Read the model definition and answer for the solid it produces. Units are mm, in the model's axes. Face numbers are marked on the shaded views. A direction names the side the tool comes from. Give positions to 0.01 mm unless a question says otherwise; leave off trailing zeros. Write each loop counter-clockwise with the first axis right and the second up, starting at its lowest first coordinate (ties: lowest second). Pieces come first, ordered by that corner, then holes. Notation, with made-up numbers: (-26, 4) - (-4, 4) arc R23 ccw to (-4, 28) - close; hole circle Ø6 at (-5.75, 2.5). An arc over 180 degrees is marked (long way). Answer as a JSON object with one key per item and string values. Group by question number.
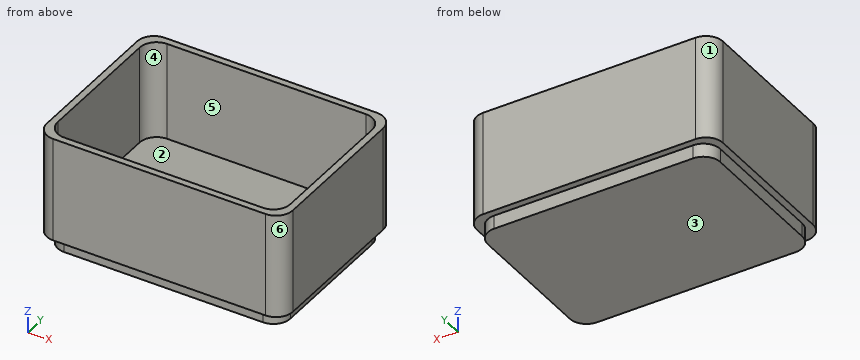
```python
from build123d import *

# Parameters (mm, degrees)
F1_DEPTH = 6
F2_DEPTH = 35
F3_DEPTH = 4


with BuildPart() as f1:
    # F0 (on Top) → F1 (new body)
    with BuildSketch(Plane.XY):
        with BuildLine():
            Line((31.5, 26.5), (-31.5, 26.5))
            ThreePointArc((-31.5, 26.5), (-35.0355339059, 25.0355339059), (-36.5, 21.5))
            Line((-36.5, 21.5), (-36.5, -21.5))
            ThreePointArc((-36.5, -21.5), (-35.0355339059, -25.0355339059), (-31.5, -26.5))
            Line((-31.5, -26.5), (31.5, -26.5))
            ThreePointArc((31.5, -26.5), (35.0355339059, -25.0355339059), (36.5, -21.5))
            Line((36.5, -21.5), (36.5, 21.5))
            ThreePointArc((36.5, 21.5), (35.0355339059, 25.0355339059), (31.5, 26.5))
        make_face()
        with BuildLine():
            ThreePointArc((-34.5, 19.5), (-33.0355339059, 23.0355339059), (-29.5, 24.5))
            Line((-29.5, 24.5), (29.5, 24.5))
            ThreePointArc((29.5, 24.5), (33.0355339059, 23.0355339059), (34.5, 19.5))
            Line((34.5, 19.5), (34.5, -19.5))
            ThreePointArc((34.5, -19.5), (33.0355339059, -23.0355339059), (29.5, -24.5))
            Line((29.5, -24.5), (-29.5, -24.5))
            ThreePointArc((-29.5, -24.5), (-33.0355339059, -23.0355339059), (-34.5, -19.5))
            Line((-34.5, -19.5), (-34.5, 19.5))
        make_face(mode=Mode.SUBTRACT)
        with BuildLine():
            Line((29.5, 24.5), (-29.5, 24.5))
            ThreePointArc((-29.5, 24.5), (-33.0355339059, 23.0355339059), (-34.5, 19.5))
            Line((-34.5, 19.5), (-34.5, -19.5))
            ThreePointArc((-34.5, -19.5), (-33.0355339059, -23.0355339059), (-29.5, -24.5))
            Line((-29.5, -24.5), (29.5, -24.5))
            ThreePointArc((29.5, -24.5), (33.0355339059, -23.0355339059), (34.5, -19.5))
            Line((34.5, -19.5), (34.5, 19.5))
            ThreePointArc((34.5, 19.5), (33.0355339059, 23.0355339059), (29.5, 24.5))
        make_face()
    extrude(amount=F1_DEPTH)

    # F0 (on Top) → F2 (join)
    with BuildSketch(Plane.XY):
        with BuildLine():
            Line((31.5, 26.5), (-31.5, 26.5))
            ThreePointArc((-31.5, 26.5), (-35.0355339059, 25.0355339059), (-36.5, 21.5))
            Line((-36.5, 21.5), (-36.5, -21.5))
            ThreePointArc((-36.5, -21.5), (-35.0355339059, -25.0355339059), (-31.5, -26.5))
            Line((-31.5, -26.5), (31.5, -26.5))
            ThreePointArc((31.5, -26.5), (35.0355339059, -25.0355339059), (36.5, -21.5))
            Line((36.5, -21.5), (36.5, 21.5))
            ThreePointArc((36.5, 21.5), (35.0355339059, 25.0355339059), (31.5, 26.5))
        make_face()
        with BuildLine():
            ThreePointArc((-34.5, 19.5), (-33.0355339059, 23.0355339059), (-29.5, 24.5))
            Line((-29.5, 24.5), (29.5, 24.5))
            ThreePointArc((29.5, 24.5), (33.0355339059, 23.0355339059), (34.5, 19.5))
            Line((34.5, 19.5), (34.5, -19.5))
            ThreePointArc((34.5, -19.5), (33.0355339059, -23.0355339059), (29.5, -24.5))
            Line((29.5, -24.5), (-29.5, -24.5))
            ThreePointArc((-29.5, -24.5), (-33.0355339059, -23.0355339059), (-34.5, -19.5))
            Line((-34.5, -19.5), (-34.5, 19.5))
        make_face(mode=Mode.SUBTRACT)
    extrude(amount=F2_DEPTH)

    # F0 (on Top) → F3 (cut)
    with BuildSketch(Plane.XY):
        with BuildLine():
            Line((31.5, 26.5), (-31.5, 26.5))
            ThreePointArc((-31.5, 26.5), (-35.0355339059, 25.0355339059), (-36.5, 21.5))
            Line((-36.5, 21.5), (-36.5, -21.5))
            ThreePointArc((-36.5, -21.5), (-35.0355339059, -25.0355339059), (-31.5, -26.5))
            Line((-31.5, -26.5), (31.5, -26.5))
            ThreePointArc((31.5, -26.5), (35.0355339059, -25.0355339059), (36.5, -21.5))
            Line((36.5, -21.5), (36.5, 21.5))
            ThreePointArc((36.5, 21.5), (35.0355339059, 25.0355339059), (31.5, 26.5))
        make_face()
        with BuildLine():
            ThreePointArc((-34.5, 19.5), (-33.0355339059, 23.0355339059), (-29.5, 24.5))
            Line((-29.5, 24.5), (29.5, 24.5))
            ThreePointArc((29.5, 24.5), (33.0355339059, 23.0355339059), (34.5, 19.5))
            Line((34.5, 19.5), (34.5, -19.5))
            ThreePointArc((34.5, -19.5), (33.0355339059, -23.0355339059), (29.5, -24.5))
            Line((29.5, -24.5), (-29.5, -24.5))
            ThreePointArc((-29.5, -24.5), (-33.0355339059, -23.0355339059), (-34.5, -19.5))
            Line((-34.5, -19.5), (-34.5, 19.5))
        make_face(mode=Mode.SUBTRACT)
    extrude(amount=F3_DEPTH, mode=Mode.SUBTRACT)


solid = f1.part
```
1) Find section C-C, the plane x = -5. Write down the section's boundary in (y, z).
2) Which of the six approach directions +Z, -Z, +X, -X, +Y, -Y give full straight-line access (tool end or side, diameter ignored) to the marked faces 5 and 6?
3) Find section A-A, the plane y = 10. Write down the section's boundary in (x, z), and give its area (3 significant figures).
4) Find the intervals of material crossed by line 1 (X direction, y = 7, z = 16.5); line 2 (Y direction, x = -19, z = 15.5); line 3 (Z direction, x = -2, y = 3.5), in increasing order. Write a range as [from, to].
5) Flat-ended cylindrical pins translate along their axes: pin 1 Ø24.5 at (x, y) = (15, 7.5) entering from +Z; pin 2 Ø2 at (y, z) = (-4.5, 1) entering from -X; pin 3 Ø3 at (y, z) = (-5, 1.5) entering from +X. Find the tip coordinate at first contact, or state that the pin passes through.
6) Find section B-B, the plane z = 22. Write down the section's boundary in (x, y), and give its area (3 significant figures).
7) For a pull along X with two mould halves and no side action, classify the marked faces 1, 2, 3 and 4 as released by +X, released by -X, zero draft, split by the parting line, or undercut.
Values follow:
{
 "1": {"outline": "(-26.5, 4) - (-24.5, 4) - (-24.5, 0) - (24.5, 0) - (24.5, 4) - (26.5, 4) - (26.5, 35) - (24.5, 35) - (24.5, 6) - (-24.5, 6) - (-24.5, 35) - (-26.5, 35) - close"},
 "2": {"face 5": "+Z", "face 6": "+Z, -Z, +X, -Y"},
 "3": {"outline": "(-36.5, 4) - (-34.5, 4) - (-34.5, 0) - (34.5, 0) - (34.5, 4) - (36.5, 4) - (36.5, 35) - (34.5, 35) - (34.5, 6) - (-34.5, 6) - (-34.5, 35) - (-36.5, 35) - close", "area": "538 mm2"},
 "4": {"line 1": "x = [-36.5, -34.5], [34.5, 36.5]", "line 2": "y = [-26.5, -24.5], [24.5, 26.5]", "line 3": "z = [0, 6]"},
 "5": {"pin 1": "stops at z = 6", "pin 2": "stops at x = -34.5", "pin 3": "stops at x = 34.5"},
 "6": {"outline": "(-36.5, -21.5) arc R5 ccw to (-31.5, -26.5) - (31.5, -26.5) arc R5 ccw to (36.5, -21.5) - (36.5, 21.5) arc R5 ccw to (31.5, 26.5) - (-31.5, 26.5) arc R5 ccw to (-36.5, 21.5) - close; hole (-34.5, -19.5) arc R5 ccw to (-29.5, -24.5) - (29.5, -24.5) arc R5 ccw to (34.5, -19.5) - (34.5, 19.5) arc R5 ccw to (29.5, 24.5) - (-29.5, 24.5) arc R5 ccw to (-34.5, 19.5) - close", "area": "488 mm2"},
 "7": {"face 1": "released by -X", "face 2": "undercut", "face 3": "zero draft", "face 4": "undercut"}
}
